from build123d import *

# Parameters (mm, degrees)
SKETCH1_W               = 76.2
SKETCH1_H               = 50.8
BOSS_EXTRUDE1_DEPTH     = 50.8
CUT_EXTRUDE1_DEPTH      = 1
CUT_EXTRUDE1_DEPTH_BACK = 22.86
CUT_EXTRUDE2_DEPTH      = 77.2
SKETCH6_R               = 6.35
CUT_EXTRUDE3_DEPTH      = 51.8


with BuildPart() as part:
    # Sketch1 → Boss-Extrude1 (new body)
    with BuildSketch(Plane.XY):
        with Locations((38.1, 25.4)):
            Rectangle(SKETCH1_W, SKETCH1_H)
    extrude(amount=BOSS_EXTRUDE1_DEPTH)

    # Sketch2 → Cut-Extrude1 (cut, two sides)
    with BuildSketch(Plane(origin=(0, 50.8, 0), x_dir=(1, 0, 0), z_dir=(0, 1, 0))) as cut_extrude1_sk:
        Polygon((76.2, -12.7), (50.8, -50.8), (76.2, -50.8), align=None)
        Polygon((0, -12.7), (0, -50.8), (25.4, -50.8), align=None)
    extrude(amount=CUT_EXTRUDE1_DEPTH, mode=Mode.SUBTRACT)
    extrude(cut_extrude1_sk.sketch, amount=-CUT_EXTRUDE1_DEPTH_BACK, mode=Mode.SUBTRACT)

    # Sketch3 → Cut-Extrude2 (cut, through all)
    with BuildSketch(Plane(origin=(76.2, 0, 0), x_dir=(0, 0, -1), z_dir=(1, 0, 0))):
        Polygon((-12.7, 50.8), (-50.8, 40.591135768), (-50.8, 50.8), align=None)
    extrude(amount=-CUT_EXTRUDE2_DEPTH, mode=Mode.SUBTRACT)

    # Sketch6 → Cut-Extrude3 (cut, through all)
    with BuildSketch(Plane.XY.offset(50.8)):
        with Locations((38.1, 12.7)):
            Circle(SKETCH6_R)
    extrude(amount=-CUT_EXTRUDE3_DEPTH, mode=Mode.SUBTRACT)


solid = part.part
Source: CAD feature listing. Evaluate the final solid. Frame: model axes, mm. A direction names the side the tool comes from. Give positions to 0.01 mm unless a question says otherwise; leave off trailing zeros. Order: outer loops, then holes, each group sorted by start corner. A loop starts at its lowest first (then second) coordinate and runs counter-clockwise, first axis right, second up. Notation, with made-up numbers: (48.25, 3.25) -> (67.25, 3.25) arc R18 cw to (67.25, 10.25) -> close; hole circle Ø6 at (-10.5, 73.25). An arc over 180 degrees is marked (long way). Use a Markdown table: item, result.
1) Reachability of faces 4 (the flat face through (38, 0, 25)), 5 (the flat face through (12.88, 36.99, 32.02)), 6 (the flat face through (64, 37, 31)) from +Z, -Z, +X, -X, +Y, -Y: full face, straight path, thin tool, end or side. Return the list, or none.
Answer list:
| item | result |
|---|---|
| face 4 | +Z, -Z, +X, -X, -Y |
| face 5 | +Z, -X, +Y |
| face 6 | +Z, +X, +Y |
2) Contact query for flat-ended pins moving along their axis: P1, Ø20.5, axis at x = 66, z = 36.5, coming from the +Y side; P2, Ø4, axis at y = 44.5, z = 18, coming from the -X side; P3, Ø8, axis at y = 38.5, z = 17, coming from the +X side. Output: stop coordinate, or through.
Answer list:
| item | result |
|---|---|
| P1 | y = 47.17 |
| P2 | x = 2.2 |
| P3 | x = 76 |
3) Section query D-D, the plane x = 27.5. Return the cut outline in (y, z).
Answer list:
| item | result |
|---|---|
| outline | (0, 0) -> (50.8, 0) -> (50.8, 12.7) -> (40.59, 50.8) -> (0, 50.8) -> close |
4) Mould query, pull axis X, two halves, no side actions, for faces 1 (the cylindrical face through (31.756, 12.979, 25.756)), 2 (the flat face through (38, 50.8, 6)), 3 (the flat face through (76.2, 19, 19)). Classes: +X half, -X half, draft (parallel to the pull), parting line (faces both ways), or undercut.
Answer list:
| item | result |
|---|---|
| face 1 | undercut |
| face 2 | draft |
| face 3 | +X half |
5) Section query C-C, the plane z = 45. Return the cut outline in (x, y), then the cut area to 3 significant figures.
Answer list:
| item | result |
|---|---|
| outline | (0, 0) -> (76.2, 0) -> (76.2, 27.94) -> (54.67, 27.94) -> (54.67, 42.15) -> (21.53, 42.15) -> (21.53, 27.94) -> (0, 27.94) -> close; hole circle Ø12.7 at (38.1, 12.7) |
| area | 2,470 mm² |
6) Section query B-B, the plane x = 38.1. Return the cut outline in (y, z).
Answer list:
| item | result |
|---|---|
| outline | (0, 0) -> (6.35, 0) -> (6.35, 50.8) -> (0, 50.8) -> close; (19.05, 0) -> (50.8, 0) -> (50.8, 12.7) -> (40.59, 50.8) -> (19.05, 50.8) -> close |
7) Section query A-A, the plane y = 12.7. Return the cut outline in (x, z), then the cut area to 3 significant figures.
Answer list:
| item | result |
|---|---|
| outline | (0, 0) -> (31.75, 0) -> (31.75, 50.8) -> (0, 50.8) -> close; (44.45, 0) -> (76.2, 0) -> (76.2, 50.8) -> (44.45, 50.8) -> close |
| area | 3,230 mm² |
8) Ray query, line 1 along Y through (x, z) = (4.5, 44); line 2 along Y through (x, z) = (33.5, 34); line 3 along Y through (x, z) = (38.1, 15.5). Return the intervals inside material, ascending. Write a range as [from, to].
Answer list:
| item | result |
|---|---|
| line 1 | [0, 27.94] |
| line 2 | [0, 8.32], [17.08, 45.09] |
| line 3 | [0, 6.35], [19.05, 50.05] |
